```python
from build123d import *

# Parameters (mm, degrees)
F0_W          = 1066.8
F0_H          = 1066.8
F1_DEPTH      = 355.6
F2_W          = 1092.2
F2_H          = 381
F3_DEPTH      = 19.05
F4_R          = 6.35
F5_W          = 489.0489578247
F5_H          = 210.7685804367
F5_H_2        = 396.8377411366
F6_DEPTH      = 330.2
F7_W          = 482.892036438
F7_H          = 204.61165905
F7_W_2        = 482.9529523849
F7_H_2        = 390.7417356968
F8_DEPTH      = 330.2
F8_DEPTH_BACK = 6.35


with BuildPart() as f1:
    # F0 (on Front) → F1 (new body)
    with BuildSketch(Plane.XZ):
        with Locations((-533.4, 533.4)):
            Rectangle(F0_W, F0_H)
    extrude(amount=F1_DEPTH)

    # F2 (on face) → F3 (join)
    with BuildSketch(Plane.XY.offset(1066.8)):
        with Locations((-533.4, -177.8)):
            Rectangle(F2_W, F2_H)
    extrude(amount=F3_DEPTH)

    # F4
    f4_edges = [f1.edges().sort_by_distance(p)[0] for p in [
        (-533.4, 12.7, 1085.85),
        (-1079.5, -177.8, 1085.85),
        (-533.4, -368.3, 1085.85),
        (12.7, -177.8, 1085.85),
    ]]
    fillet(f4_edges, radius=F4_R)

    # F5 (on face) → F6 (cut)
    with BuildSketch(Plane.XZ.offset(355.6)):
        with Locations((-793.9267158508, 923.8921999931)):
            Rectangle(F5_W, F5_H)
        with Locations((-275.7667158508, 923.8921999931)):
            Rectangle(F5_W, F5_H)
        with Locations((-276.6835210876, 677.9517097816)):
            Rectangle(F5_W, F5_H)
        with Locations((-794.8435210876, 677.9517097816)):
            Rectangle(F5_W, F5_H)
        with Locations((-794.8435210876, 343.4552997351)):
            Rectangle(F5_W, F5_H_2)
        with Locations((-276.6835210876, 343.4552997351)):
            Rectangle(F5_W, F5_H_2)
    extrude(amount=-F6_DEPTH, mode=Mode.SUBTRACT)

    # F7 (on face) → F8 (join, two sides)
    with BuildSketch(Plane.XZ.offset(355.6)) as f8_sk:
        with Locations((-793.9267158508, 923.8921999931)):
            Rectangle(F7_W, F7_H)
        with Locations((-793.9267158508, 678.5281999931)):
            Rectangle(F7_W, F7_H)
        with Locations((-276.0715158508, 923.8921999931)):
            Rectangle(F7_W, F7_H)
        with Locations((-276.0715158508, 678.5281999931)):
            Rectangle(F7_W, F7_H)
        with Locations((-794.8435210876, 343.4552997351)):
            Rectangle(F7_W_2, F7_H_2)
        with Locations((-276.6835210876, 343.4552997351)):
            Rectangle(F7_W_2, F7_H_2)
    extrude(amount=-F8_DEPTH)
    extrude(f8_sk.sketch, amount=F8_DEPTH_BACK)


solid = f1.part
```
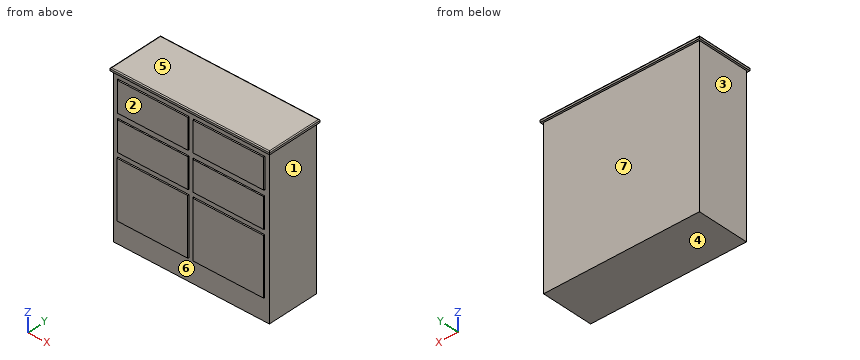
Verification items for the finished model (mm, model axes). Face numbers are marked on the shaded views. A direction names the side the tool comes from. Coordinates: 2 decimals unless noted, no trailing zeros. Order: outer loops, then holes, each group sorted by start corner. A loop starts at its lowest first (then second) coordinate and runs counter-clockwise, first axis right, second up. Notation, with made-up numbers: (-1.5, -2) - (28.5, -2) arc R13 cw to (28.5, 17) - close; hole circle Ø4 at (26, 71.5). An arc over 180 degrees is marked (long way). Return JSON: item names as keys, results as strings.
(1) Go/stop test with flat-tipped pins: pin 1 (3 mm diameter, centred on x = -579, z = 891.5, fed in from -Y); pin 2 (5 mm diameter, centred on y = -122.5, z = 958, fed in from -X); pin 3 (10 mm diameter, centred on y = -326.5, z = 337.5, fed in from +X). Record where each tip stops, or that it passes through.
Filled sheet:
{"pin 1": "stops at y = -361.95", "pin 2": "stops at x = -1066.8", "pin 3": "stops at x = 0"}
(2) Section check A-A, the plane z = 239.5. Record the cut outline in (x, y).
Filled sheet:
{"outline": "(-1066.8, -355.6) - (-1039.37, -355.6) - (-1039.37, -25.4) - (-1036.32, -25.4) - (-1036.32, -361.95) - (-553.37, -361.95) - (-553.37, -25.4) - (-550.32, -25.4) - (-550.32, -355.6) - (-521.21, -355.6) - (-521.21, -25.4) - (-518.16, -25.4) - (-518.16, -361.95) - (-35.21, -361.95) - (-35.21, -25.4) - (-32.16, -25.4) - (-32.16, -355.6) - (0, -355.6) - (0, 0) - (-1066.8, 0) - close"}
(3) Section check C-C, the plane y = -249. Give the number of separate pieces and of enclosed holes in the cut face, and give its area (3 significant figures).
Filled sheet:
{"separate pieces": "7", "enclosed holes": "6", "area": "1,130,000 mm^2"}
(4) Section check D-D, the plane z = 109. Record the cut outline in (x, y), and give its area (3 significant figures).
Filled sheet:
{"outline": "(-1066.8, -355.6) - (0, -355.6) - (0, 0) - (-1066.8, 0) - close", "area": "379,000 mm^2"}
(5) Access from +Z, -Z, +X, -X, +Y, -Y to the whole of each face (thin tool, end or side, straight path). Record for the marked faces 1, 2, 3 and 4.
Filled sheet:
{"face 1": "-Z, +X, +Y, -Y", "face 2": "-Z, +X, -X, -Y", "face 3": "-Z, -X, +Y, -Y", "face 4": "-Z, +X, -X, +Y, -Y"}
(6) Mould release check, pull along Z, two halves, no side actions. Record for the marked faces 5, 6 and 7: pulls with the +Z half, pulls with the -Z half, needs draft (parallel to the pull), parting line crosses it, or undercut.
Filled sheet:
{"face 5": "pulls with the +Z half", "face 6": "undercut", "face 7": "needs draft"}
(7) Thickness scan on line 1 along X through (y, z) = (-97, 652); line 2 along X through (y, z) = (-319, 284); line 3 along X through (y, z) = (-173, 147). Record the ranges inside material, lowest first.
Filled sheet:
{"line 1": "x = -1066.8 to -1039.37, -1035.37 to -552.48, -550.32 to -521.21, -517.52 to -34.63, -32.16 to 0", "line 2": "x = -1066.8 to -1039.37, -1036.32 to -553.37, -550.32 to -521.21, -518.16 to -35.21, -32.16 to 0", "line 3": "x = -1066.8 to -1039.37, -550.32 to -521.21, -32.16 to 0"}
